```python
from build123d import *

# Parameters (mm, degrees)
BOSS_EXTRUDE1_DEPTH = 4


with BuildPart() as part:
    # Sketch1 → Boss-Extrude1 (new body)
    with BuildSketch(Plane.XY):
        with BuildLine():
            Line((0, 0), (3.5, 0))
            ThreePointArc((3.5, 0), (6.5, 3), (9.5, 0))
            Line((9.5, 0), (14, 0))
            Line((14, 0), (14, -4))
            Line((14, -4), (24, -4))
            Line((24, -4), (24, 0))
            Line((24, 0), (31.049410002, 0))
            ThreePointArc((31.049410002, 0), (32.903799592, 1.250840974), (32.438642701, 3.438760754))
            Line((32.438642701, 3.438760754), (3.3892327, 31.488170756))
            ThreePointArc((3.3892327, 31.488170756), (1.218483973, 31.890396884), (0, 30.049410002))
            Line((0, 30.049410002), (0, 23))
            Line((0, 23), (-4, 23))
            Line((-4, 23), (-4, 13))
            Line((-4, 13), (0, 13))
            Line((0, 13), (0, 0))
        make_face()
    extrude(amount=BOSS_EXTRUDE1_DEPTH)


solid = part.part
```
The model under review builds one solid part; all positions refer to its coordinate system, in mm. A direction names the side the tool comes from. Round coordinates to 2 decimals unless told otherwise and drop trailing zeros. Order: outer loops, then holes, each group sorted by start corner. A loop starts at its lowest first (then second) coordinate and runs counter-clockwise, first axis right, second up. Notation, with made-up numbers: (27, 60.5) - (46, 60.5) arc R23 ccw to (46, 89.5) - close; hole circle Ø3 at (-36.75, -23.5). An arc over 180 degrees is marked (long way). Answer in a Markdown table with one row per item.
(1) Take a section at B-B on y = 22.5. Write out the cut boundary in (x, z).
Result set:
| item | result |
|---|---|
| outline | (-4, 0) - (12.7, 0) - (12.7, 4) - (-4, 4) - close |
(2) Take a section at A-A on z = 3.1. Write out the cut boundary in (x, y), plus the area to 3 significant figures.
Result set:
| item | result |
|---|---|
| outline | (-4, 13) - (0, 13) - (0, 0) - (3.5, 0) arc R3 cw to (9.5, 0) - (14, 0) - (14, -4) - (24, -4) - (24, 0) - (31.05, 0) arc R2 ccw to (32.44, 3.44) - (3.39, 31.49) arc R2 ccw to (0, 30.05) - (0, 23) - (-4, 23) - close |
| area | 682 mm2 |
(3) Machinability: for faces 1 (the face through (-2, 13, 2)), 2 (the face through (32.89, 1.22, 1.97)), 3 (the face through (10, 10, 0)), 4 (the face through (24, -2, 2)), 5 (the face through (-2, 23, 2)), which of the approach directions +Z, -Z, +X, -X, +Y, -Y give a long, thin tool a straight path to every point of the face, cutting with its end or side? Answer none if there is none.
Result set:
| item | result |
|---|---|
| face 1 | +Z, -Z, -X, -Y |
| face 2 | +Z, -Z, +X |
| face 3 | -Z, +X, -X, +Y, -Y |
| face 4 | +Z, -Z, +X, -Y |
| face 5 | +Z, -Z, -X, +Y |
(4) For line 1 (Y direction, x = -0.5, z = 2.95); line 2 (Y direction, x = 20, z = 3.75); line 3 (X direction, y = 30.5, z = 1.25), list the stretches that pass through material, from the lowest coordinate up. Write a range as from..to.
Result set:
| item | result |
|---|---|
| line 1 | y = 13..23 |
| line 2 | y = -4..15.45 |
| line 3 | x = 0.05..4.41 |
(5) Mouldability with a two-part tool opening along X and no side actions: class faces 6 (the face through (6.4, 3, 2)), 7 (the face through (14, -2, 2)), 8 (the face through (27, 0, 2)) as released by +X, released by -X, zero draft, split by the parting line, or undercut.
Result set:
| item | result |
|---|---|
| face 6 | undercut |
| face 7 | released by -X |
| face 8 | zero draft |
(6) Take a section at C-C on x = 23.5. Write out the cut boundary in (y, z), plus the area to 3 significant figures.
Result set:
| item | result |
|---|---|
| outline | (-4, 0) - (12.07, 0) - (12.07, 4) - (-4, 4) - close |
| area | 64.3 mm2 |
(7) Clearance check with flat-ended pins moving along their axes: P1, Ø1.5, axis at x = 0, z = 1.5, coming from the -Y side; P2, Ø1.2, axis at y = -2, z = 1, coming from the +X side; P3, Ø1.2, axis at y = 25, z = 3, coming from the -X side. State where each tip first meets the part, or that it passes through.
Result set:
| item | result |
|---|---|
| P1 | stops at y = 0 |
| P2 | stops at x = 24 |
| P3 | stops at x = 0 |
